```python
from build123d import *

# Parameters (mm, degrees)
F0_R     = 16.7005
F0_R_2   = 13.3223
F1_DEPTH = 152.4
F3_R     = 28.470245
F4_DEPTH = 25.4


with BuildPart() as f1:
    # F0 (on Front) → F1 (new body, symmetric)
    with BuildSketch(Plane.XZ):
        Circle(F0_R)
        Circle(F0_R_2, mode=Mode.SUBTRACT)
    extrude(amount=F1_DEPTH, both=True)


with BuildPart() as f4:
    # F3 (on Right) → F4 (new body)
    with BuildSketch(Plane.YZ):
        with Locations((44.697168, 50.904491)):
            Circle(F3_R)
    extrude(amount=F4_DEPTH)


solid = f1.part
```
Can you work these out from the model? Positions are in its coordinate system, mm. Coordinates: 2 decimals unless noted, no trailing zeros. Loops run counter-clockwise (first coordinate to the right, second up) from the corner with the lowest first, then second, coordinate; pieces in that order, holes last. Notation, with made-up numbers: (68, -38) - (87, -38) arc R34 ccw to (87, -1) - close; hole circle Ø6 at (-30, 50). An arc over 180 degrees is marked (long way). Answer as CSV lines item,"result". Start each with the question number.
1) Suppose I cut it at B-B (z = 0). Please give me the cut outline in (x, y), plus the area to 3 significant figures.
2) For pin 1 (3 mm diameter, centred on x = 13, y = -19, fed in from +Z); pin 2 (3 mm diameter, centred on x = 11, y = -56, fed in from -Z); pin 3 (10 mm diameter, centred on y = 71, z = 10, fed in from -X), each with a flat end and sliding along its axis, tell me the tip position at first contact or that it passes through.
3) Suppose I cut it at C-C (y = 123). Please give me the cut outline in (x, z).
4) Thinking about a two-plate mould opening in Z: for faces 1 (the cylindrical face through (12.707, 2.134, 4.002)), 2 (the flat face through (-1, -152.4, -14)), 3 (the cylindrical face through (-3.62, -2.134, -16.303)), which applies, pulls with the +Z half, pulls with the -Z half, needs draft (parallel to the pull), parting line crosses it, or undercut?
5) Suppose I cut it at A-A (x = 0). Please give me the cut outline in (y, z), plus the area to 3 significant figures.
6) I need wall thicknesses on line 1 (X direction, y = 55.5, z = -1); line 2 (Z direction, x = 0, y = -21); line 3 (Z direction, x = 10, y = -107). Which ranges of each line are inside material? Lowest first, please. Write a range as from..to.
Check result:
1,outline,"(-16.7, -152.4) - (-13.32, -152.4) - (-13.32, 152.4) - (-16.7, 152.4) - close; (13.32, -152.4) - (16.7, -152.4) - (16.7, 152.4) - (13.32, 152.4) - close"
1,area,"2,060 mm²"
2,pin 1,"stops at z = 12.11"
2,pin 2,"stops at z = -13.74"
2,pin 3,"stops at x = -15.93"
3,outline,"circle Ø33.4 at (0, 0); hole circle Ø26.64 at (0, 0)"
4,face 1,"undercut"
4,face 2,"needs draft"
4,face 3,"parting line crosses it"
5,outline,"(-152.4, -16.7) - (152.4, -16.7) - (152.4, -13.32) - (-152.4, -13.32) - close; (-152.4, 13.32) - (152.4, 13.32) - (152.4, 16.7) - (-152.4, 16.7) - close"
5,area,"2,060 mm²"
6,line 1,"x = -16.67..-13.28, 13.28..16.67"
6,line 2,"z = -16.7..-13.32, 13.32..16.7"
6,line 3,"z = -13.38..-8.8, 8.8..13.38"
